Can you work these out from the drawing? Everything is in mm from the part's minimum corner. Give positions to 0.01 mm unless a question says otherwise; leave off trailing zeros. Write each loop counter-clockwise with the first axis right and the second up, starting at its lowest first coordinate (ties: lowest second). Pieces come first, ordered by that corner, then holes. Notation, with made-up numbers: (-20.5, 74.5) -> (15.5, 74.5) arc R22 ccw to (15.5, 107.5) -> close; hole circle Ø7 at (52, 23.5). An arc over 180 degrees is marked (long way). Use one line per item in the form item = value.
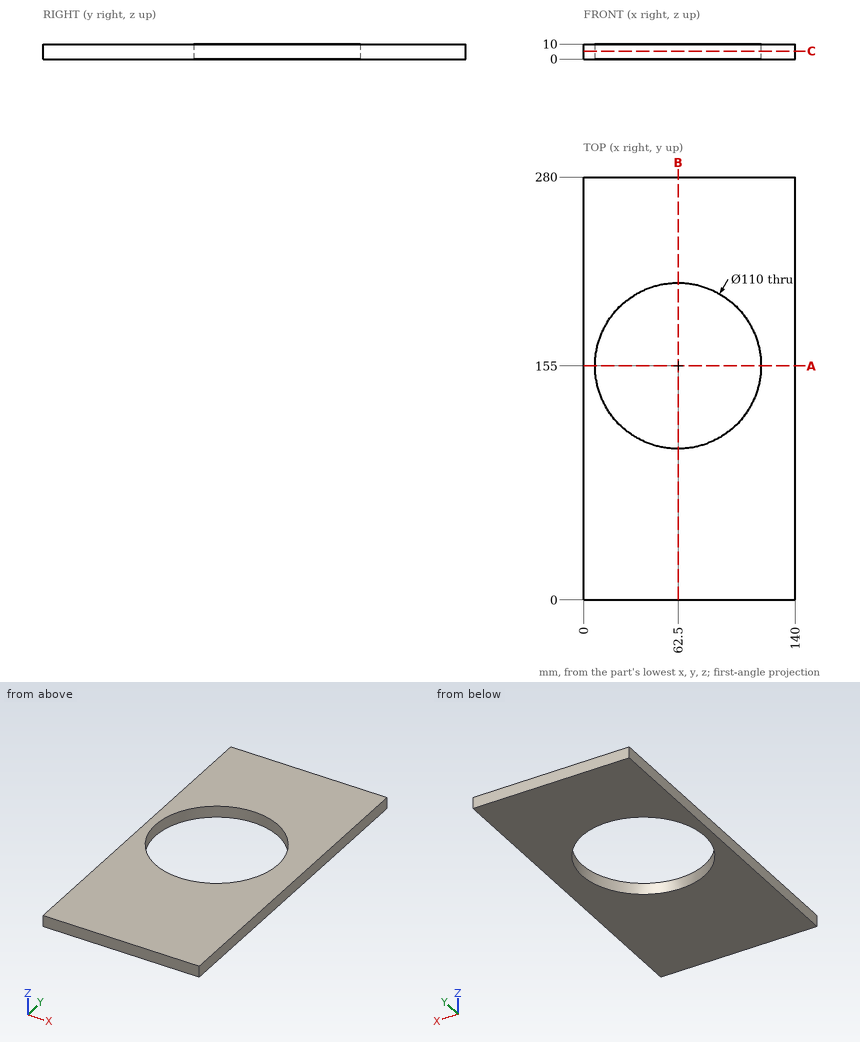
Q1. I want a section at B-B, the plane x = 62.5. Write out the boundary of the cut face in (y, z), and give its area (3 significant figures).
Result set:
outline = (0, 0) -> (100, 0) -> (100, 10) -> (0, 10) -> close; (210, 0) -> (280, 0) -> (280, 10) -> (210, 10) -> close
area = 1,700 mm2
Q2. If I drill on line 1 along Y through (x, z) = (62.5, 2.25); line 2 along X through (y, z) = (155, 3); line 3 along Y through (x, z) = (101.5, 1.5), over which ranges is the centre line in solid material (lowest first)? Write a range as from..to.
Result set:
line_1 = 0..100, 210..280
line_2 = 0..7.5, 117.5..140
line_3 = 0..116.22, 193.78..280
Q3. I want a section at C-C, the plane z = 5.25. Write out the boundary of the cut face in (x, y), and give its area (3 significant figures).
Result set:
outline = (0, 0) -> (140, 0) -> (140, 280) -> (0, 280) -> close; hole circle Ø110 at (62.5, 155)
area = 29,700 mm2
Q4. I want a section at A-A, the plane y = 155. Write out the boundary of the cut face in (x, z).
Result set:
outline = (0, 0) -> (7.5, 0) -> (7.5, 10) -> (0, 10) -> close; (117.5, 0) -> (140, 0) -> (140, 10) -> (117.5, 10) -> close
